```python
from build123d import *

# Parameters (mm, degrees)
SKETCH1_W           = 150
SKETCH1_H           = 150
BOSS_EXTRUDE1_DEPTH = 59
SKETCH2_W           = 130
SKETCH2_H           = 130
CUT_EXTRUDE1_DEPTH  = 60
SKETCH9_R           = 1.4
CUT_EXTRUDE4_DEPTH  = 10
CIRPATTERN1_COUNT   = 3
CIRPATTERN1_ANGLE   = 180
SKETCH10_W          = 130
SKETCH10_H          = 96.398295943
CUT_EXTRUDE6_DEPTH  = 60
SKETCH11_R          = 2.5
CUT_EXTRUDE7_DEPTH  = 151


with BuildPart() as part:
    # Sketch1 → Boss-Extrude1 (new body)
    with BuildSketch(Plane(origin=(0, 0, 0), x_dir=(1, 0, 0), z_dir=(0, 1, 0))):
        Rectangle(SKETCH1_W, SKETCH1_H)
    extrude(amount=-BOSS_EXTRUDE1_DEPTH)

    # Sketch2 → Cut-Extrude1 (cut, through all)
    with BuildSketch(Plane(origin=(0, 0, 0), x_dir=(1, 0, 0), z_dir=(0, 1, 0))):
        Rectangle(SKETCH2_W, SKETCH2_H)
    extrude(amount=-CUT_EXTRUDE1_DEPTH, mode=Mode.SUBTRACT)

    # Sketch9 → Cut-Extrude4 (cut)
    with BuildSketch(Plane.ZY.offset(75)):
        with Locations((-6.1, -7.25)):
            Circle(SKETCH9_R)
        with Locations((6.1, -7.25)):
            Circle(SKETCH9_R)
        with Locations((6.1, -15.25)):
            Circle(SKETCH9_R)
        with Locations((-6.1, -15.25)):
            Circle(SKETCH9_R)
    cut_extrude4 = extrude(amount=-CUT_EXTRUDE4_DEPTH, mode=Mode.SUBTRACT)

    # CirPattern1: Cut-Extrude4 ×3 about axis
    cirpattern1_axis = Axis((0, 0, 0), (0, 1, 0))
    for i in range(1, CIRPATTERN1_COUNT):
        add(cut_extrude4.rotate(cirpattern1_axis, i * CIRPATTERN1_ANGLE / (CIRPATTERN1_COUNT - 1)), mode=Mode.SUBTRACT)

    # Sketch10 → Cut-Extrude6 (cut, through all)
    with BuildSketch(Plane(origin=(0, 0, 0), x_dir=(1, 0, 0), z_dir=(0, 1, 0))):
        with Locations((0, 113.199147972)):
            Rectangle(SKETCH10_W, SKETCH10_H)
    extrude(amount=-CUT_EXTRUDE6_DEPTH, mode=Mode.SUBTRACT)

    # Sketch11 → Cut-Extrude7 (cut, through all)
    with BuildSketch(Plane(origin=(75, 0, 0), x_dir=(0, 0, -1), z_dir=(1, 0, 0))):
        with Locations((0, -49.5)):
            Circle(SKETCH11_R)
    extrude(amount=-CUT_EXTRUDE7_DEPTH, mode=Mode.SUBTRACT)


solid = part.part
```
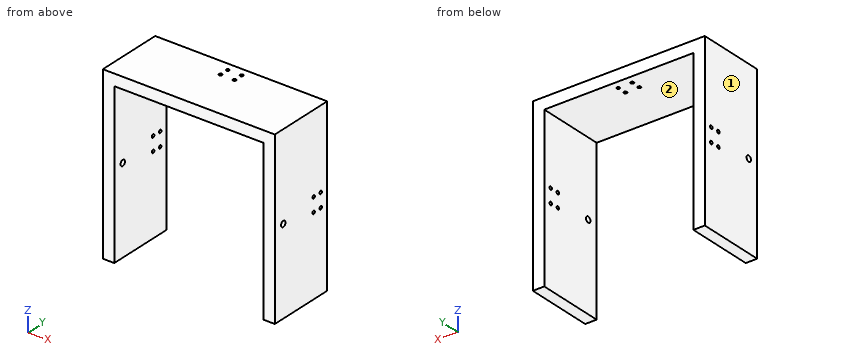
The listing builds one solid part. Answer for the finished solid, in the listing's coordinates (mm). Face numbers are marked on the shaded views. A direction names the side the tool comes from. Round coordinates to 2 decimals unless told otherwise and drop trailing zeros. Loops run counter-clockwise (first coordinate to the right, second up) from the corner with the lowest first, then second, coordinate; pieces in that order, holes last. Notation, with made-up numbers: (74.5, 27.25) -> (112.5, 27.25) arc R28 cw to (112.5, 64.25) -> close; hole circle Ø3 at (78, -11). An arc over 180 degrees is marked (long way). Use one line per item in the form item = value.
1. The part is cut by section D-D on x = 0.5. Determine the outline of the cut face in (y, z).
Answer key:
outline = (-59, 65) -> (0, 65) -> (0, 75) -> (-59, 75) -> close
2. A tool of negligible diameter and unlimited length cuts with its end or side. For the marked faces 1 and 2, from which of +Z, -Z, +X, -X, +Y, -Y can it reach the whole face along a straight path? Write none if from no direction.
Answer key:
face_1 = +Z, -Z, -X, +Y, -Y
face_2 = -Z, +Y, -Y
3. The part is cut by section A-A on z = 0. Determine the outline of the cut face in (x, y), and give its area (3 significant figures).
Answer key:
outline = (-75, -59) -> (-65, -59) -> (-65, -52) -> (-75, -52) -> close; (-75, -47) -> (-65, -47) -> (-65, 0) -> (-75, 0) -> close; (65, -59) -> (75, -59) -> (75, -52) -> (65, -52) -> close; (65, -47) -> (75, -47) -> (75, 0) -> (65, 0) -> close
area = 1,080 mm²
4. The part is cut by section C-C on y = -42.5. Determine the outline of the cut face in (x, z).
Answer key:
outline = (-75, -75) -> (-65, -75) -> (-65, 65) -> (65, 65) -> (65, -75) -> (75, -75) -> (75, 75) -> (-75, 75) -> close
5. Find the intervals of material crossed by probe 1 along Y at (x, z) = (6.1, 73); probe 2 along Z at (x, y) = (72, -7); probe 3 along X at (y, z) = (-22, 58), in increasing order. Write a range as [from, to].
Answer key:
probe_1 = [-59, -16.65], [-13.85, -8.65], [-5.85, 0]
probe_2 = [-75, -7.48], [-4.72, 4.72], [7.48, 75]
probe_3 = [-75, -65], [65, 75]
6. The part is cut by section B-B on z = 26.5. Determine the outline of the cut face in (x, y), and give its area (3 significant figures).
Answer key:
outline = (-75, -59) -> (-65, -59) -> (-65, 0) -> (-75, 0) -> close; (65, -59) -> (75, -59) -> (75, 0) -> (65, 0) -> close
area = 1,180 mm²
7. Flat-ended cylindrical pins translate along their axes: pin 1 Ø6 at (y, z) = (-49.5, 0) entering from -X; pin 2 Ø3 at (x, y) = (6.1, -7.25) entering from -Z. Find the tip coordinate at first contact, or state that the pin passes through.
Answer key:
pin_1 = -75
pin_2 = 65
